Check sheet for the modelled part. Datum: model origin and axes. Units: mm. A direction names the side the tool comes from. Round coordinates to 2 decimals unless told otherwise and drop trailing zeros. Write each loop counter-clockwise with the first axis right and the second up, starting at its lowest first coordinate (ties: lowest second). Pieces come first, ordered by that corner, then holes. Notation, with made-up numbers: (85.5, 89) - (108.5, 89) arc R18 cw to (108.5, 95) - close; hole circle Ø6 at (-32.5, 22). An arc over 180 degrees is marked (long way). Answer as a JSON object with one key per item and string values. Group by question number.
Item 1: Set-up check for faces 1 (the flat face through (1, 12, 4.075)), 2 (the flat face through (-5.355, 4, -6)), 3 (the flat face through (-16.87, 1.5, -0.05)), 4 (the flat face through (-13.555, 4, 0)): record each of +Z, -Z, +X, -X, +Y, -Y from which the full face is reachable in a straight line by a thin tool's end or side.
Item 2: Release check for a two-part mould opening along Z. For faces 5 (the flat face through (-14.055, 3, 0)), 6 (the flat face through (5.075, 7, -7)), 7 (the flat face through (0, 3.37, 0)), 8 (the flat face through (10, 4, -6.545)) record: pulls with the +Z half, pulls with the -Z half, needs draft (parallel to the pull), parting line crosses it, or undercut.
Item 3: Gauge pin test, flat ends, axial feed: P1, Ø1.1, axis at x = -16, y = 1.5, coming from the -Z side (3 decimals); P2, Ø9, axis at y = 13, z = 1, coming from the -X side; P3, Ø2, axis at x = -2, z = 4.5, coming from the +Y side. Record the tip position at first contact, or that the pin passes through.
Item 4: Sectioned sample at C-C on z = 0. Count the separate pieces of the cut face and the enclosed holes in it, plus the area to 3 significant figures.
Item 5: Sectioned sample at A-A on x = 19.5. Record the boundary of the cut face in (y, z), plus the area to 3 significant figures.
Item 6: Sectioned sample at D-D on x = -15.5. Record the boundary of the cut face in (y, z) (3 decimals).
Item 7: Sectioned sample at B-B on y = 2.25. Record the boundary of the cut face in (x, z) (3 decimals), plus the area to 3 significant figures.
Item 8: Thickness scan on line 1 (X direction, y = 1.1, z = 0) (3 decimals); line 2 (Y direction, x = -3, z = -2.25); line 3 (X direction, y = 20.25, z = -2.25). Record the ranges inside material, lowest first.
```python
from build123d import *

# Parameters (mm, degrees)
BOSS_EXTRUDE1_DEPTH     = 7.2
SKETCH2_R               = 1.61
BOSS_EXTRUDE2_DEPTH     = 1.5
BOSS_EXTRUDE3_DEPTH     = 0.7
BOSS_EXTRUDE4_DEPTH     = 14.4
BOSS_EXTRUDE4_TAPER     = 0.5
SKETCH5_W               = 10.15
SKETCH5_H               = 8.4
BOSS_EXTRUDE5_DEPTH     = 10.12
SKETCH6_W               = 10.15
SKETCH6_H               = 5.5
BOSS_EXTRUDE6_DEPTH     = 6.35
BOSS_EXTRUDE7_DEPTH     = 4.22
CUT_EXTRUDE1_DEPTH      = 7.544999991
CUT_EXTRUDE1_DEPTH_BACK = 10.824999991
SKETCH9_W               = 27.11
SKETCH9_H               = 10.549999982
BOSS_EXTRUDE8_DEPTH     = 1.2


with BuildPart() as part:
    # Sketch1 → Boss-Extrude1 (new body)
    with BuildSketch(Plane(origin=(0, 0, 0), x_dir=(1, 0, 0), z_dir=(0, 1, 0))):
        Polygon((-14.055, 5.774999991), (-5.355, 5.774999991), (-5.355, 6.544999991), (-14.825, 6.544999991), (-14.825, -6.544999991), (14.825, -6.544999991), (14.825, 6.544999991), (5.355, 6.544999991), (5.355, 5.774999991), (14.055, 5.774999991), (14.055, -5.774999991), (-14.055, -5.774999991), align=None)
    extrude(amount=BOSS_EXTRUDE1_DEPTH)

    # Sketch2 → Boss-Extrude2 (add)
    with BuildSketch(Plane(origin=(0, 0, 0), x_dir=(1, 0, 0), z_dir=(0, 1, 0))):
        with BuildLine():
            Line((18.64, 3.735), (14.825, 3.735))
            Line((14.825, 3.735), (14.825, -3.735))
            Line((14.825, -3.735), (18.64, -3.735))
            ThreePointArc((18.64, -3.735), (22.375, 0), (18.64, 3.735))
        make_face()
        with Locations((18.64, 0)):
            Circle(SKETCH2_R, mode=Mode.SUBTRACT)
        with BuildLine():
            Line((-14.825, 3.735), (-14.825, -3.735))
            Line((-14.825, -3.735), (-18.64, -3.735))
            ThreePointArc((-18.64, -3.735), (-22.375, 0), (-18.64, 3.735))
            Line((-18.64, 3.735), (-14.825, 3.735))
        make_face()
        with Locations((-18.64, 0)):
            Circle(SKETCH2_R, mode=Mode.SUBTRACT)
    extrude(amount=BOSS_EXTRUDE2_DEPTH)

    # Sketch3 → Boss-Extrude3 (add)
    with BuildSketch(Plane(origin=(0, 7.2, 0), x_dir=(1, 0, 0), z_dir=(0, 1, 0))):
        Polygon((-14.825, -6.544999991), (14.825, -6.544999991), (14.825, 6.544999991), (5.355, 6.544999991), (5.355, 4.324999991), (-5.355, 4.324999991), (-5.355, 6.544999991), (-14.825, 6.544999991), align=None)
    extrude(amount=-BOSS_EXTRUDE3_DEPTH)

    # Sketch4 → Boss-Extrude4 (add)
    with BuildSketch(Plane(origin=(0, 7.2, 0), x_dir=(1, 0, 0), z_dir=(0, 1, 0))):
        with BuildLine():
            Line((-14.325, -6), (-4.825, -6))
            ThreePointArc((-4.825, -6), (-4.471446609, -5.853553391), (-4.325, -5.5))
            Line((-4.325, -5.5), (-4.325, 5.5))
            ThreePointArc((-4.325, 5.5), (-4.471446609, 5.853553391), (-4.825, 6))
            Line((-4.825, 6), (-14.325, 6))
            ThreePointArc((-14.325, 6), (-14.678553391, 5.853553391), (-14.825, 5.5))
            Line((-14.825, 5.5), (-14.825, -5.5))
            ThreePointArc((-14.825, -5.5), (-14.678553391, -5.853553391), (-14.325, -6))
        make_face()
        with BuildLine():
            Line((-13.625, -4.58), (-5.525, -4.58))
            ThreePointArc((-5.525, -4.58), (-5.171446609, -4.433553391), (-5.025, -4.08))
            Line((-5.025, -4.08), (-5.025, 4.08))
            ThreePointArc((-5.025, 4.08), (-5.171446609, 4.433553391), (-5.525, 4.58))
            Line((-5.525, 4.58), (-13.625, 4.58))
            ThreePointArc((-13.625, 4.58), (-13.978553391, 4.433553391), (-14.125, 4.08))
            Line((-14.125, 4.08), (-14.125, -4.08))
            ThreePointArc((-14.125, -4.08), (-13.978553391, -4.433553391), (-13.625, -4.58))
        make_face(mode=Mode.SUBTRACT)
        with BuildLine():
            Line((6.325, -6), (14.325, -6))
            ThreePointArc((14.325, -6), (14.678553391, -5.853553391), (14.825, -5.5))
            Line((14.825, -5.5), (14.825, 5.5))
            ThreePointArc((14.825, 5.5), (14.678553391, 5.853553391), (14.325, 6))
            Line((14.325, 6), (6.325, 6))
            ThreePointArc((6.325, 6), (5.971446609, 5.853553391), (5.825, 5.5))
            Line((5.825, 5.5), (5.825, -5.5))
            ThreePointArc((5.825, -5.5), (5.971446609, -5.853553391), (6.325, -6))
        make_face()
        with BuildLine():
            Line((6.955, -4.6), (13.695, -4.6))
            ThreePointArc((13.695, -4.6), (14.048553391, -4.453553391), (14.195, -4.1))
            Line((14.195, -4.1), (14.195, 4.1))
            ThreePointArc((14.195, 4.1), (14.048553391, 4.453553391), (13.695, 4.6))
            Line((13.695, 4.6), (6.955, 4.6))
            ThreePointArc((6.955, 4.6), (6.601446609, 4.453553391), (6.455, 4.1))
            Line((6.455, 4.1), (6.455, -4.1))
            ThreePointArc((6.455, -4.1), (6.601446609, -4.453553391), (6.955, -4.6))
        make_face(mode=Mode.SUBTRACT)
    extrude(amount=BOSS_EXTRUDE4_DEPTH, taper=BOSS_EXTRUDE4_TAPER)

    # Sketch5 → Boss-Extrude5 (add)
    with BuildSketch(Plane(origin=(0, 7.2, 0), x_dir=(1, 0, 0), z_dir=(0, 1, 0))):
        with Locations((0.75, 0.124999991)):
            Rectangle(SKETCH5_W, SKETCH5_H)
    extrude(amount=BOSS_EXTRUDE5_DEPTH)

    # Sketch6 → Boss-Extrude6 (add)
    with BuildSketch(Plane(origin=(0, 3.37, 0), x_dir=(1, 0, 0), z_dir=(0, 1, 0))):
        with Locations((0, 7.074999991)):
            Rectangle(SKETCH6_W, SKETCH6_H)
    extrude(amount=BOSS_EXTRUDE6_DEPTH)

    # Sketch7 → Boss-Extrude7 (add)
    with BuildSketch(Plane(origin=(0, 1.5, 0), x_dir=(1, 0, 0), z_dir=(0, 1, 0))):
        with BuildLine():
            Line((-14.825, 3.735), (-16.625, 3.735))
            ThreePointArc((-16.625, 3.735), (-15.518302355, 2.690023234), (-14.825, 1.335))
            Line((-14.825, 1.335), (-14.825, 3.735))
        make_face()
        with BuildLine():
            Line((-14.825, -3.735), (-14.825, -1.335))
            ThreePointArc((-14.825, -1.335), (-15.518302355, -2.690023234), (-16.625, -3.735))
            Line((-16.625, -3.735), (-14.825, -3.735))
        make_face()
        with BuildLine():
            Line((14.825, -3.735), (16.625, -3.735))
            ThreePointArc((16.625, -3.735), (15.518302355, -2.690023234), (14.825, -1.335))
            Line((14.825, -1.335), (14.825, -3.735))
        make_face()
        with BuildLine():
            Line((14.825, 3.735), (14.825, 1.335))
            ThreePointArc((14.825, 1.335), (15.518302355, 2.690023234), (16.625, 3.735))
            Line((16.625, 3.735), (14.825, 3.735))
        make_face()
    extrude(amount=BOSS_EXTRUDE7_DEPTH)

    # Sketch8 → Cut-Extrude1 (cut, two sides)
    with BuildSketch(Plane.XY) as cut_extrude1_sk:
        Polygon((-14.825, 5.72), (-16.625, 3.92), (-16.625, 5.72), align=None)
        Polygon((14.825, 5.72), (16.625, 3.92), (16.625, 5.72), align=None)
    extrude(amount=CUT_EXTRUDE1_DEPTH, mode=Mode.SUBTRACT)
    extrude(cut_extrude1_sk.sketch, amount=-CUT_EXTRUDE1_DEPTH_BACK, mode=Mode.SUBTRACT)

    # Sketch9 → Boss-Extrude8 (add)
    with BuildSketch(Plane.XZ.offset(-3.37)):
        Rectangle(SKETCH9_W, SKETCH9_H)
    extrude(amount=-BOSS_EXTRUDE8_DEPTH)


solid = part.part
```
Completed:
{
 "1": {"face 1": "+Z, +Y", "face 2": "-Z", "face 3": "-X, +Y", "face 4": "-Y"},
 "2": {"face 5": "undercut", "face 6": "needs draft", "face 7": "undercut", "face 8": "pulls with the -Z half"},
 "3": {"P1": "z = -3.735", "P2": "x = -14.81", "P3": "y = 17.32"},
 "4": {"separate pieces": "4", "enclosed holes": "0", "area": "210 mm²"},
 "5": {"outline": "(0, -3.63) - (1.5, -3.63) - (1.5, -1.36) - (0, -1.36) - close; (0, 1.36) - (1.5, 1.36) - (1.5, 3.63) - (0, 3.63) - close", "area": "6.82 mm²"},
 "6": {"outline": "(0, -3.735) - (5.045, -3.735) - (5.045, -2.665) - (1.5, -2.665) - (1.5, 2.665) - (5.045, 2.665) - (5.045, 3.735) - (0, 3.735) - close"},
 "7": {"outline": "(-16.625, -3.735) - (-14.825, -3.735) - (-14.825, -6.545) - (-5.355, -6.545) - (-5.355, -5.775) - (-14.055, -5.775) - (-14.055, 5.775) - (14.055, 5.775) - (14.055, -5.775) - (5.355, -5.775) - (5.355, -6.545) - (14.825, -6.545) - (14.825, -3.735) - (16.625, -3.735) arc R4.483 cw to (14.825, -1.335) - (14.825, 1.335) arc R4.483 cw to (16.625, 3.735) - (14.825, 3.735) - (14.825, 6.545) - (-14.825, 6.545) - (-14.825, 3.735) - (-16.625, 3.735) arc R4.483 cw to (-14.825, 1.335) - (-14.825, -1.335) arc R4.483 cw to start", "area": "61.8 mm²"},
 "8": {"line 1": "-22.375 to -20.25, -17.03 to -14.055, 14.055 to 17.03, 20.25 to 22.375", "line 2": "3.37 to 4.57, 6.5 to 17.32", "line 3": "-14.71 to -14.24, -4.91 to -4.44, 5.94 to 6.34, 14.31 to 14.71"}
}
